from build123d import *

# Parameters (mm, degrees)
BOSS_EXTRUDE1_DEPTH = 2.778125
SKETCH3_R           = 1.5
SKETCH3_R_2         = 1.499997
CUT_EXTRUDE2_DEPTH  = 2.778125


with BuildPart() as part:
    # Sketch1 → Boss-Extrude1 (new body)
    with BuildSketch(Plane.XY):
        Polygon((-111.521875, 114.3), (-114.3, 114.3), (-114.3, 101.6), (-111.521875, 101.6), (-111.521875, 88.9), (-114.3, 88.9), (-114.3, 76.2), (-111.521875, 76.2), (-111.521875, 63.5), (-114.3, 63.5), (-114.3, 50.8), (-111.521875, 50.8), (-111.521875, 38.1), (-114.3, 38.1), (-114.3, 25.4), (-111.521875, 25.4), (-111.521875, 12.7), (-114.3, 12.7), (-114.3, 0), (-111.521875, 0), (-111.521875, -12.7), (-114.3, -12.7), (-114.3, -25.4), (-111.521875, -25.4), (-111.521875, -38.1), (-114.3, -38.1), (-114.3, -50.8), (-111.521875, -50.8), (-111.521875, -63.5), (-114.3, -63.5), (-114.3, -76.2), (-111.521875, -76.2), (-111.521875, -88.9), (-114.3, -88.9), (-114.3, -101.6), (-111.521875, -101.6), (-111.521875, -114.3), (-114.3, -114.3), (-114.3, -127), (-95.25, -127), (-95.25, -133.35), (-57.15, -133.35), (-57.15, -127), (-19.05, -127), (-19.05, -133.35), (19.05, -133.35), (19.05, -127), (57.15, -127), (57.15, -133.35), (95.25, -133.35), (95.25, -127), (114.3, -127), (114.3, -114.3), (111.521875, -114.3), (111.521875, -101.6), (114.3, -101.6), (114.3, -88.9), (111.521875, -88.9), (111.521875, -76.2), (114.3, -76.2), (114.3, -63.5), (111.521875, -63.5), (111.521875, -50.8), (114.3, -50.8), (114.3, -38.1), (111.521875, -38.1), (111.521875, -25.4), (114.3, -25.4), (114.3, -12.7), (111.521875, -12.7), (111.521875, 0), (114.3, 0), (114.3, 12.7), (111.521875, 12.7), (111.521875, 25.4), (114.3, 25.4), (114.3, 38.1), (111.521875, 38.1), (111.521875, 50.8), (114.3, 50.8), (114.3, 63.5), (111.521875, 63.5), (111.521875, 76.2), (114.3, 76.2), (114.3, 88.9), (111.521875, 88.9), (111.521875, 101.6), (114.3, 101.6), (114.3, 114.3), (111.521875, 114.3), (111.521875, 127), (-111.521875, 127), align=None)
    extrude(amount=BOSS_EXTRUDE1_DEPTH)

    # Sketch3 → Cut-Extrude2 (cut)
    with BuildSketch(Plane(origin=(0, 0, 0), x_dir=(-1, 0, 0), z_dir=(0, 0, -1))):
        with Locations((-95.25, 112)):
            Circle(SKETCH3_R)
        with Locations((-95.25, 96.25)):
            Circle(SKETCH3_R_2)
        with Locations((95.25, 96.25)):
            Circle(SKETCH3_R_2)
        with Locations((95.25, 112)):
            Circle(SKETCH3_R)
    extrude(amount=-CUT_EXTRUDE2_DEPTH, mode=Mode.SUBTRACT)


solid = part.part
Could you check a few things on this model? Use its own coordinates, in mm. Give positions to 0.01 mm unless a question says otherwise; leave off trailing zeros. Write each loop counter-clockwise with the first axis right and the second up, starting at its lowest first coordinate (ties: lowest second). Pieces come first, ordered by that corner, then holes. Notation, with made-up numbers: (83, 87) -> (94, 87) arc R18 ccw to (94, 91) -> close; hole circle Ø1 at (42.5, 22.25). An arc over 180 degrees is marked (long way). Answer as CSV lines item,"result". Start each with the question number.
(1) If we section it at C-C, the plane x = -46.5: Write out the boundary of the cut face in (y, z).
(2) If we section it at A-A, the plane z = 1: Give the number of separate pieces and of enclosed holes in the cut face, and give its area (3 significant figures).
(3) If we section it at B-B, the plane y = -35: Write out the boundary of the cut face in (x, z).
(4) I'm going to push flat-ended pins straight in: pin 1 Ø1.4 at (y, z) = (-131, 1.5) entering from -X; pin 2 Ø3.5 at (x, y) = (-95.25, 112) entering from +Z; pin 3 Ø1.4 at (y, z) = (71, 1) entering from -X; pin 4 Ø0.8 at (y, z) = (95.5, 2) entering from +X. Where does each tip first touch, or does it pass through?
(5) Please list where these lines run through material, in increasing order: line 1 (X direction, y = 96.25, z = 1.1); line 2 (X direction, y = 112, z = 0.8); line 3 (Y direction, x = 23, z = 2.6).
Answer list:
1,outline,"(-127, 0) -> (127, 0) -> (127, 2.78) -> (-127, 2.78) -> close"
2,separate pieces,"1"
2,enclosed holes,"4"
2,area,"58,100 mm^2"
3,outline,"(-111.52, 0) -> (111.52, 0) -> (111.52, 2.78) -> (-111.52, 2.78) -> close"
4,pin 1,"x = -95.25"
4,pin 2,"z = 2.78"
4,pin 3,"x = -111.52"
4,pin 4,"x = 111.52"
5,line 1,"-111.52 to -96.75, -93.75 to 93.75, 96.75 to 111.52"
5,line 2,"-114.3 to -96.75, -93.75 to 93.75, 96.75 to 114.3"
5,line 3,"-127 to 127"
